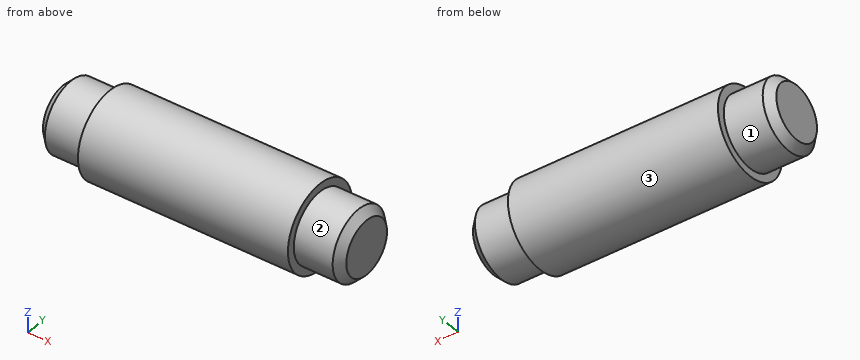
Autodesk Inventor part; units mm, degrees
ref_plane "YZ Plane" through (0, 0, 0) normal (1, 0, 0) x (0, 1, 0)
ref_plane "XZ Plane" through (0, 0, 0) normal (0, 1, 0) x (-1, 0, 0)
ref_plane "XY Plane" through (0, 0, 0) normal (0, 0, 1) x (1, 0, 0)
sketch "Sketch1" plane through (0, 0, 0) normal (0, 0, 1) x (1, 0, 0)
  line L0 (0, 0) -> (78, 0)
  line L1 (78, 0) -> (78, 8.95)
  line L2 (78, 8.95) -> (66, 8.95)
  line L3 (66, 8.95) -> (66, 10.95)
  line L4 (66, 10.95) -> (12, 10.95)
  line L5 (12, 10.95) -> (12, 8.95)
  line L6 (12, 8.95) -> (0, 8.95)
  line L7 (0, 8.95) -> (0, 0)
  dimension "d0" = 78
  dimension "d1" = 8.95
  dimension "d2" = 12
  dimension "d3" = 2
  dimension "d4" = 54
  dimension "d5" = 2
revolve "Revolution1" add sketch "Sketch1" angle 360 about axis through (0, 0, 0) along (1, 0, 0)
chamfer "Chamfer1" distance 2 angle 45 1 edges at (78, -8.95, 0) measured on face at (78, 1.5348, -1.8062)
chamfer "Chamfer2" distance 2 angle 45 1 edges at (0, -8.95, 0) measured on face at (0, -2.9314, 2.1504)
properties part number "axle" material "Steel, Carbon"
Here's how the part is built. I have some questions about the finished solid (model axes, mm). Face numbers are marked on the shaded views. A direction names the side the tool comes from. Coordinates: 2 decimals unless noted, no trailing zeros. Order: outer loops, then holes, each group sorted by start corner. A loop starts at its lowest first (then second) coordinate and runs counter-clockwise, first axis right, second up.
1) Will these pins go through, and if not, where does the flat tip stop? pin 1 (5 mm diameter, centred on x = 46, z = 8.5, fed in from +Y); pin 2 (12 mm diameter, centred on x = 31.5, y = 8, fed in from +Z); pin 3 (1 mm diameter, centred on x = 41.5, z = 1, fed in from -Y).
2) Imagine slicing it at D-D on x = 52.5. List the corners of the cut face in (y, z) for me, and give its area (3 significant figures).
3) Which directions (+Z, -Z, +X, -X, +Y, -Y) give clear straight access to the entire face, cutting with the end or side of a thin tool? Please do the marked faces 1, 2 and 3.
4) I need wall thicknesses on line 1 (X direction, y = -8.25, z = 3.75); line 2 (Z direction, x = 11, y = 5.75); line 3 (Y direction, x = 50, z = 7). Which ranges of each line are inside material? Lowest first, please.
5) Imagine slicing it at C-C on x = 6. List the corners of the cut face in (y, z) for me, and give its area (3 significant figures).
6) Imagine slicing it at A-A on z = 0. List the corners of the cut face in (x, y) for me.
Response values:
1. pin 1: stops at y = 9.16
1. pin 2: stops at z = 10.77
1. pin 3: stops at y = -10.94
2. outline: circle Ø21.9 at (0, 0)
2. area: 377 mm2
3. face 1: -X
3. face 2: +X
3. face 3: +X, -X
4. line 1: x = 12 to 66
4. line 2: z = -6.86 to 6.86
4. line 3: y = -8.42 to 8.42
5. outline: circle Ø17.9 at (0, 0)
5. area: 252 mm2
6. outline: (0, -6.95) - (2, -8.95) - (12, -8.95) - (12, -10.95) - (66, -10.95) - (66, -8.95) - (76, -8.95) - (78, -6.95) - (78, 6.95) - (76, 8.95) - (66, 8.95) - (66, 10.95) - (12, 10.95) - (12, 8.95) - (2, 8.95) - (0, 6.95) - close
